The model under review builds one solid part; all positions refer to its coordinate system, in mm. Face numbers are marked on the shaded views. A direction names the side the tool comes from. Round coordinates to 2 decimals unless told otherwise and drop trailing zeros. Order: outer loops, then holes, each group sorted by start corner. A loop starts at its lowest first (then second) coordinate and runs counter-clockwise, first axis right, second up.
from build123d import *

# Parameters (mm, degrees)
F1_DEPTH = 22.352
F2_DEPTH = 3.175
F3_R     = 22.35199
F5_DEPTH = 9.652
F7_R     = 3.175
F8_DEPTH = 25.4
F7_R_2   = 6.35
F9_DEPTH = 3.175
F10_R    = 10.922


# Not quite as in the source:
# - a fillet or chamfer is up to 0.001 mm smaller than in the source, because OpenCascade refuses the exact size


with BuildPart() as f1:
    # F0 (on Front) → F1 (new body, symmetric)
    with BuildSketch(Plane.XZ):
        Polygon((-21.8362923991, 37.8215678842), (0, 0), (91.4245847982, 0), (91.4245847982, 9.652), (30.9725847982, 9.652), (5.5725847982, 9.652), (-13.4774152018, 42.6475678842), align=None)
    extrude(amount=F1_DEPTH, both=True)

    # F0 (on Front) → F2 (join, symmetric)
    with BuildSketch(Plane.XZ):
        Polygon((30.9725847982, 9.652), (-13.4774152018, 42.6475678842), (5.5725847982, 9.652), align=None)
    extrude(amount=F2_DEPTH, both=True)

    # F3 (radius 22.352 in the source; OpenCascade refuses exactly that, so slightly less here)
    f3_edges = [f1.edges().sort_by_distance(p)[0] for p in [
        (91.424585, 22.352, 4.826),
        (91.424585, -22.352, 4.826),
    ]]
    fillet(f3_edges, radius=F3_R)

    # F4 (on face) → F5 (cut, through all)
    with BuildSketch(Plane.XY.offset(9.652)):
        with BuildLine():
            Line((69.0725847982, 9.652), (43.6725847982, 9.652))
            ThreePointArc((43.6725847982, 9.652), (34.0205847982, 0), (43.6725847982, -9.652))
            Line((43.6725847982, -9.652), (69.0725847982, -9.652))
            ThreePointArc((69.0725847982, -9.652), (78.7245847982, 0), (69.0725847982, 9.652))
        make_face()
    extrude(amount=-F5_DEPTH, mode=Mode.SUBTRACT)

    # F7 (on face) → F8 (cut)
    with BuildSketch(Plane(origin=(8.3588771973, 0, 4.826), x_dir=(0, 1, 0), z_dir=(0.8660254038, 0, 0.5))):
        with Locations((11.43, 32.7505847982)):
            Circle(F7_R)
        with Locations((-11.43, 32.7505847982)):
            Circle(F7_R)
    extrude(amount=-F8_DEPTH, mode=Mode.SUBTRACT)

    # F7 (on face) → F9 (cut)
    with BuildSketch(Plane(origin=(8.3588771973, 0, 4.826), x_dir=(0, 1, 0), z_dir=(0.8660254038, 0, 0.5))):
        with Locations((-11.43, 32.7505847982)):
            Circle(F7_R_2)
        with Locations((-11.43, 32.7505847982)):
            Circle(F7_R, mode=Mode.SUBTRACT)
        with Locations((11.43, 32.7505847982)):
            Circle(F7_R_2)
        with Locations((11.43, 32.7505847982)):
            Circle(F7_R, mode=Mode.SUBTRACT)
    extrude(amount=-F9_DEPTH, mode=Mode.SUBTRACT)

    # F10
    f10_edges = [f1.edges().sort_by_distance(p)[0] for p in [
        (-17.656854, 22.352, 40.234568),
        (-17.656854, -22.352, 40.234568),
    ]]
    fillet(f10_edges, radius=F10_R)


solid = f1.part
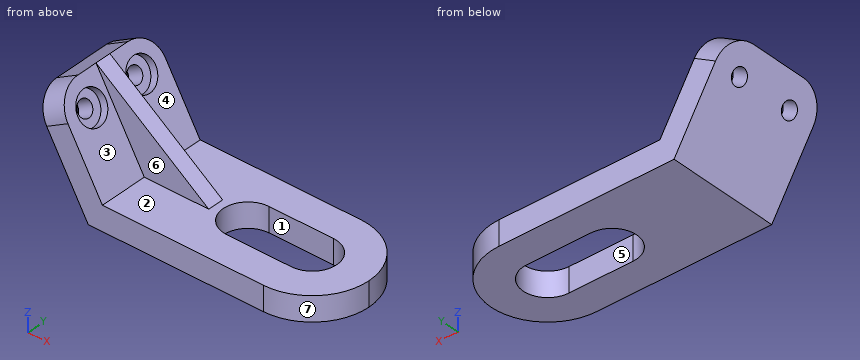
(1) Clearance check with flat-ended pins moving along their axes: P1, Ø13.5, axis at x = 64.5, y = -11, coming from the +Z side; P2, Ø16.5, axis at x = 15, z = 27, coming from the -Y side (3 decimals); P3, Ø12, axis at x = 7, y = -2.5, coming from the +Z side. State where each tip first meets the part, or that it passes through.
(2) We need section D-D (x = 15). Give the boundary of the cut face in (y, z) (3 decimals), and give its area (3 significant figures).
(3) We need section A-A (y = 13.5). Give the boundary of the cut face in (x, z), and give its area (3 significant figures).
(4) Tool access review of the marked faces 1, 2, 3 and 4: name each direction out of +Z, -Z, +X, -X, +Y, -Y from which nothing blocks a thin tool from reaching the whole face with its end or side.
(5) The part is to be moulded in two halves that separate along X. For the marked faces 5, 6 and 7, say which applies: pulls with the +X half, pulls with the -X half, needs draft (parallel to the pull), parting line crosses it, or undercut.
(6) We need section B-B (x = 41.5). Give the boundary of the cut face in (y, z).
(7) To check wall thickness, follow L1, parallel to Z at x = 18, y = -6; L2, parallel to X at y = -1, z = 6; L3, parallel to X at y = 10, z = 19.5. State the ranges of each line that lie inside material, in increasing order.
Verdict:
1. P1: stops at z = 9.65
1. P2: stops at y = -3.175
1. P3: stops at z = 31.9
2. outline: (-22.352, 0) - (22.352, 0) - (22.352, 9.652) - (3.175, 9.652) - (3.175, 21.509) - (-3.175, 21.509) - (-3.175, 9.652) - (-22.352, 9.652) - close
2. area: 507 mm2
3. outline: (-21.74, 37.65) - (-17.58, 30.45) - (-11.97, 33.69) - (-13.77, 36.8) - (-11.02, 38.39) - (-13.38, 42.48) - close; (-15.17, 26.28) - (0, 0) - (86.89, 0) - (86.89, 9.65) - (5.57, 9.65) - (-5.01, 27.99) - (-7.76, 26.4) - (-9.56, 29.52) - close
3. area: 1,140 mm2
4. face 1: +Z, -Z
4. face 2: +Z, +X
4. face 3: +Z, +X, -Y
4. face 4: +Z, +X, +Y
5. face 5: undercut
5. face 6: needs draft
5. face 7: pulls with the +X half
6. outline: (-22.35, 0) - (-9.4, 0) - (-9.4, 9.65) - (-22.35, 9.65) - close; (9.4, 0) - (22.35, 0) - (22.35, 9.65) - (9.4, 9.65) - close
7. L1: z = 0 to 9.65
7. L2: x = -3.46 to 34.07, 78.67 to 91.4
7. L3: x = -11.26 to -0.11
